Here's how the part is built. I have some questions about the finished solid (model axes, mm). A direction names the side the tool comes from. Round coordinates to 2 decimals unless told otherwise and drop trailing zeros. Order: outer loops, then holes, each group sorted by start corner. A loop starts at its lowest first (then second) coordinate and runs counter-clockwise, first axis right, second up. Notation, with made-up numbers: (63.5, 81) - (67.5, 81) arc R32 cw to (67.5, 108) - close; hole circle Ø6 at (-11.75, 86). An arc over 180 degrees is marked (long way). One line per item, written item: value.
from build123d import *

# Parameters (mm, degrees)
SKETCH1_R             = 65
BOSS_EXTRUDE1_DEPTH   = 19
SKETCH2_R             = 5
CUT_EXTRUDE1_DEPTH    = 94.866927083
SKETCH3_R             = 3.479573806
CUT_EXTRUDE2_DEPTH    = 11.750951
CIRPATTERN1_START     = 7.249049213
CIRPATTERN1_OUTLINE_R = 3.479573806
CIRPATTERN1_DEPTH     = 11.750950787


# Read off the part's stored shape, not the designer's step: CirPattern1
with BuildPart() as part:
    # Sketch1 → Boss-Extrude1 (new body)
    with BuildSketch(Plane(origin=(0, 0, 0), x_dir=(1, 0, 0), z_dir=(0, 1, 0))):
        with Locations(Location((0, 0, 0), (0, 0, 270))):
            Circle(SKETCH1_R)
    extrude(amount=BOSS_EXTRUDE1_DEPTH)

    # Sketch2 → Cut-Extrude1 (cut, through all)
    with BuildSketch(Plane(origin=(0, 0, 0), x_dir=(1, 0, 0), z_dir=(0, 1, 0))):
        with Locations(Location((0, 0, 0), (0, 0, 270))):
            Circle(SKETCH2_R)
    extrude(amount=CUT_EXTRUDE1_DEPTH, mode=Mode.SUBTRACT)

    # Sketch3 → Cut-Extrude2 (cut)
    with BuildSketch(Plane(origin=(0, 19, 0), x_dir=(1, 0, 0), z_dir=(0, 1, 0))):
        with Locations(Location((-21.40993498, 0, 0), (0, 0, 270))):
            Circle(SKETCH3_R)
    extrude(amount=-CUT_EXTRUDE2_DEPTH, mode=Mode.SUBTRACT)

    # CirPattern1 outline → CirPattern1 (cut)
    with BuildSketch(Plane(origin=(0, 0, 0), x_dir=(1, 0, 0), z_dir=(0, 1, 0)).offset(CIRPATTERN1_START)):
        with Locations((-15.139110209, -15.139110209)):
            Circle(CIRPATTERN1_OUTLINE_R)
        with Locations((-15.139110209, 15.139110209)):
            Circle(CIRPATTERN1_OUTLINE_R)
        with Locations((0, 21.40993498)):
            Circle(CIRPATTERN1_OUTLINE_R)
        with Locations((15.139110209, 15.139110209)):
            Circle(CIRPATTERN1_OUTLINE_R)
        with Locations((21.40993498, 0)):
            Circle(CIRPATTERN1_OUTLINE_R)
        with Locations((15.139110209, -15.139110209)):
            Circle(CIRPATTERN1_OUTLINE_R)
        with Locations((0, -21.40993498)):
            Circle(CIRPATTERN1_OUTLINE_R)
    extrude(amount=CIRPATTERN1_DEPTH, mode=Mode.SUBTRACT)


solid = part.part
Q1. If I drill on line 1 along X through (y, z) = (11, 0); line 2 along Z through (x, y) = (14.5, 13.25); line 3 along X through (y, z) = (1.25, 0.5), over which ranges is the centre line in solid material (lowest first)?
Results list:
line 1: -65 to -24.89, -17.93 to -5, 5 to 17.93, 24.89 to 65
line 2: -63.36 to -18.56, -11.72 to 11.72, 18.56 to 63.36
line 3: -65 to -4.97, 4.97 to 65
Q2. If we section it at B-B, the plane x = 0: Please give me the cut outline in (y, z), then the cut area to 3 significant figures.
Results list:
outline: (0, -65) - (19, -65) - (19, -24.89) - (7.25, -24.89) - (7.25, -17.93) - (19, -17.93) - (19, -5) - (0, -5) - close; (0, 5) - (19, 5) - (19, 17.93) - (7.25, 17.93) - (7.25, 24.89) - (19, 24.89) - (19, 65) - (0, 65) - close
area: 2,120 mm²
Q3. Which directions (+Z, -Z, +X, -X, +Y, -Y) give clear straight access to the entire face, cutting with the end or side of a thin tool? Please do faces 4 (the flat face through (1, 0, 14)), 5 (the flat face through (15, 7.249, 15)).
Results list:
face 4: +Z, -Z, +X, -X, -Y
face 5: +Y
Q4. We'd pull the mould along Z, two halves only. Please class faces 1 (the cylindrical face through (19.52, 9.37, 62)), 2 (the flat face through (1, 19, 14)), 3 (the flat face through (0, 7.249, 21)): released by +Z, released by -Z, zero draft, split by the parting line, or undercut.
Results list:
face 1: split by the parting line
face 2: zero draft
face 3: undercut
Q5. If we section it at A-A, the plane z = 0: Please give me the cut outline in (x, y).
Results list:
outline: (-65, 0) - (-5, 0) - (-5, 19) - (-17.93, 19) - (-17.93, 7.25) - (-24.89, 7.25) - (-24.89, 19) - (-65, 19) - close; (5, 0) - (65, 0) - (65, 19) - (24.89, 19) - (24.89, 7.25) - (17.93, 7.25) - (17.93, 19) - (5, 19) - close
Q6. If we section it at C-C, the plane y = 16: Give the number of separate pieces and of enclosed holes in the cut face, then the cut area to 3 significant figures.
Results list:
separate pieces: 1
enclosed holes: 9
area: 12,900 mm²
Q7. Will these pins go through, and if not, where does the flat tip stop? pin 1 (2 mm diameter, centred on y = 8, z = -13, fed in from +X); pin 2 (6 mm diameter, centred on y = 10, z = 0, fed in from +X); pin 3 (10 mm diameter, centred on y = 2, z = -24.5, fed in from -X).
Results list:
pin 1: x = 63.88
pin 2: x = 65
pin 3: x = -62.01
Q8. If we section it at D-D, the plane x = -14.5: Please give me the cut outline in (y, z), then the cut area to 3 significant figures.
Results list:
outline: (0, -63.36) - (19, -63.36) - (19, -18.56) - (7.25, -18.56) - (7.25, -11.72) - (19, -11.72) - (19, 11.72) - (7.25, 11.72) - (7.25, 18.56) - (19, 18.56) - (19, 63.36) - (0, 63.36) - close
area: 2,250 mm²
